from build123d import *

# Parameters (mm, degrees)
F0_R     = 12.7
F1_DEPTH = 476.25
F2_R     = 12.7
F3_DEPTH = 47.625
F4_SIZE2 = 47.625
F4_SIZE  = 5.461
F5_R     = 12.7
F6_DEPTH = 47.625
F7_SIZE2 = 5.461
F7_SIZE  = 47.625


with BuildPart() as f1:
    # F0 (on Top) → F1 (new body)
    with BuildSketch(Plane.XY):
        Circle(F0_R)
    extrude(amount=F1_DEPTH)

    # F2 (on face) → F3 (join)
    with BuildSketch(Plane.XY.offset(476.25)):
        Circle(F2_R)
    extrude(amount=F3_DEPTH)

    # F4
    f4_edges = [f1.edges().sort_by_distance(p)[0] for p in [
        (-12.7, 0, 523.875),
    ]]
    f4_side = f1.faces().sort_by_distance((0, 0, 523.875))[0]
    chamfer(f4_edges, length=F4_SIZE, length2=F4_SIZE2, reference=f4_side)

    # F5 (on face) → F6 (join)
    with BuildSketch(Plane(origin=(0, 0, 0), x_dir=(1, 0, 0), z_dir=(0, 0, -1))):
        Circle(F5_R)
    extrude(amount=F6_DEPTH)

    # F7
    f7_edges = [f1.edges().sort_by_distance(p)[0] for p in [
        (-12.7, 0, -47.625),
    ]]
    f7_side = f1.faces().sort_by_distance((-12.7, 0, 214.3125))[0]
    chamfer(f7_edges, length=F7_SIZE, length2=F7_SIZE2, reference=f7_side)


solid = f1.part
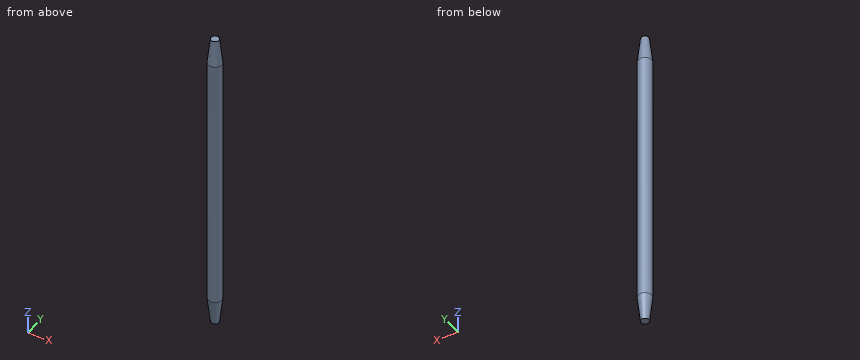
The listing builds one solid part. Answer for the finished solid, in the listing's coordinates (mm). Give positions to 0.01 mm unless a question says otherwise; leave off trailing zeros. Order: outer loops, then holes, each group sorted by start corner. A loop starts at its lowest first (then second) coordinate and runs counter-clockwise, first axis right, second up. Notation, with made-up numbers: (-29.5, -8.75) - (-23.5, -8.75) arc R15 ccw to (-23.5, -2.75) - close; hole circle Ø7 at (70, 52.25). An arc over 180 degrees is marked (long way). One line per item, written item: value. Start each with the question number.
1) A cutting plane is placed at C-C on z = 48.5. Give the vertices of the cut face in (x, y).
2) A cutting plane is placed at A-A on x = 0. Give the vertices of the cut face in (y, z) (3 decimals), then the cut area to 3 significant figures.
3) Find the intervals of material crossed by L1, parallel to X at y = 0.25, z = 98; L2, parallel to Y at x = 10, z = 479; L3, parallel to Y at x = 1.25, z = 174, in increasing order.
4) Given pin 1 Ø2 at (y, z) = (-4.5, 337) entering from +X; pin 2 Ø4 at (x, y) = (-1.5, -8.5) entering from -Z (3 decimals); pin 3 Ø8 at (x, z) = (8, 354.5) entering from +Y; pin 4 Ø12 at (y, z) = (9, 38) entering from +X, each flat-ended and moving along its own axis, determine where each tip first touches the part or whether it passes through.
Answer sheet:
1. outline: circle Ø25.4 at (0, 0)
2. outline: (-12.7, 0) - (-7.239, -47.625) - (7.239, -47.625) - (12.7, 0) - (12.7, 476.25) - (7.239, 523.875) - (-7.239, 523.875) - (-12.7, 476.25) - close
2. area: 14,000 mm2
3. L1: x = -12.7 to 12.7
3. L2: y = -7.31 to 7.31
3. L3: y = -12.64 to 12.64
4. pin 1: stops at x = 12.21
4. pin 2: stops at z = -47.625
4. pin 3: stops at y = 12.05
4. pin 4: stops at x = 12.34
